Source: CAD feature listing. Evaluate the final solid. Frame: model axes, mm. A direction names the side the tool comes from. Coordinates: 2 decimals unless noted, no trailing zeros. Write each loop counter-clockwise with the first axis right and the second up, starting at its lowest first coordinate (ties: lowest second). Pieces come first, ordered by that corner, then holes. Notation, with made-up numbers: (83, -8.75) - (139, -8.75) arc R31 ccw to (139, 21.25) - close; hole circle Ø7 at (28, -32.5). An arc over 180 degrees is marked (long way). One line per question, with ' | ' between items.
Autodesk Inventor part; units mm, degrees
ref_plane "YZ Plane" through (0, 0, 0) normal (1, 0, 0) x (0, 1, 0)
ref_plane "XZ Plane" through (0, 0, 0) normal (0, 1, 0) x (-1, 0, 0)
ref_plane "XY Plane" through (0, 0, 0) normal (0, 0, 1) x (1, 0, 0)
ref_plane "Plano de trabalho1" through (0, -45, 0) normal (0, 0, 1) x (1, 0, 0)
sketch "Esboço1" plane through (0, -45, 0) normal (0, 0, 1) x (1, 0, 0)
  arc A0 (5.5, 37.5) -> (7.5, 39.5) centre (5.5, 39.5) ccw
  line L0 (7.5, 39.5) -> (7.5, 50.5)
  arc A1 (7.5, 50.5) -> (5.5, 52.5) centre (5.5, 50.5) ccw
  line L1 (5.5, 52.5) -> (-5.5, 52.5)
  arc A2 (-5.5, 52.5) -> (-7.5, 50.5) centre (-5.5, 50.5) ccw
  line L2 (-7.5, 50.5) -> (-7.5, 39.5)
  arc A3 (-7.5, 39.5) -> (-5.5, 37.5) centre (-5.5, 39.5) ccw
  line L3 (-5.5, 37.5) -> (5.5, 37.5)
  circle A4 centre (0, 45) radius 2.1
  arc A5 (-7.5, -5.5) -> (-5.5, -7.5) centre (-5.5, -5.5) ccw
  line L4 (-5.5, -7.5) -> (5.5, -7.5)
  arc A6 (5.5, -7.5) -> (7.5, -5.5) centre (5.5, -5.5) ccw
  line L5 (7.5, -5.5) -> (7.5, 5.5)
  arc A7 (7.5, 5.5) -> (5.5, 7.5) centre (5.5, 5.5) ccw
  line L6 (5.5, 7.5) -> (-5.5, 7.5)
  arc A8 (-5.5, 7.5) -> (-7.5, 5.5) centre (-5.5, 5.5) ccw
  line L7 (-7.5, 5.5) -> (-7.5, -5.5)
  circle A9 centre (0, 0) radius 2.1
  line L8 (7.5, 39.5) -> (7.5, 5.5)
  line L9 (-7.5, 39.5) -> (-7.5, 5.5)
extrude "Extrusão1" add sketch "Esboço1" along normal blind 4
sketch "Esboço2" plane through (0, -45, 4) normal (0, 0, 1) x (1, 0, 0)
  line L0 (7.5, -5.5) -> (7.5, 50.5)
  line L1 (-7.5, 50.5) -> (-7.5, -5.5)
  line L2 (7.5, 24) -> (-7.5, 24)
  line L3 (-7.5, 24) -> (-7.5, 21)
  line L4 (-7.5, 21) -> (7.5, 21)
  line L5 (7.5, 21) -> (7.5, 24)
  line L6 (5.5, 52.5) -> (-5.5, 52.5)
  line L7 (-5.5, -7.5) -> (5.5, -7.5)
  circle A0 centre (0, 32) radius 2.1
  circle A1 centre (0, 13) radius 2.1
  point P0 (0, 45)
  point P1 (7.5, 21)
  dimension "d4" = 28.5
  dimension "d5" = 28.5
  dimension "d6" = 3
  dimension "d7" = 4.2
  dimension "d8" = 4.2
  dimension "d9" = 8
  dimension "d10" = 8
extrude "Extrusão2" cut sketch "Esboço2" against normal blind 1.5
sketch "Esboço3" plane through (0, -13, 2.5) normal (0, 0, 1) x (1, 0, 0)
  circle A0 centre (0, 0) radius 2.1
  circle A1 centre (0, -19) radius 2.1
  point P0 (0, 13)
extrude "Extrusão3" cut sketch "Esboço3" against normal blind 10
fillet "Arredondamento1" radius 1.5 2 edges at (0, -21, 2.5) (0, -24, 2.5)
equation "\"d5\" = d4"
equation "\"d10\" = d9"
properties part number "suporte_termopar_al"
Item 1: Access query for faces 5 (the face through (0, -7, 4)), 6 (the face through (0.11, -23.57, 2.95)). Directions: +Z, -Z, +X, -X, +Y, -Y. A direction counts if a zero-diameter tool reaches every point of the face in a straight line with its end or side. Return the directions, or none.
Check sheet entries:
face 5: +Z, +X, -X, +Y, -Y | face 6: +Z, +X, -X
Item 2: Pin query (flat end, axial travel): pin 1 Ø5 at (x, y) = (0, -45) entering from -Z; pin 2 Ø2.5 at (x, y) = (0, -32) entering from -Z. Return the tip coordinate at first contact, or that it passes through.
Check sheet entries:
pin 1: z = 0 | pin 2: through
Item 3: Cut plane A-A on x = 0. State how many separate pieces and enclosed holes the cut face has, and give its area (3 significant figures).
Check sheet entries:
separate pieces: 5 | enclosed holes: 0 | area: 169 mm²
Item 4: Cut plane B-B on y = -45. Return loops of the section in (x, z).
Check sheet entries:
outline: (-7.5, 0) - (-2.1, 0) - (-2.1, 4) - (-7.5, 4) - close; (2.1, 0) - (7.5, 0) - (7.5, 4) - (2.1, 4) - close
Item 5: Ray query, line 1 along Y through (x, z) = (0, 2.3); line 2 along Y through (x, z) = (-6.25, 3.2); line 3 along Y through (x, z) = (-0.5, 3.85). Return the intervals inside material, ascending. Write a range as [from, to].
Check sheet entries:
line 1: [-52.5, -47.1], [-42.9, -34.1], [-29.9, -15.1], [-10.9, -2.1], [2.1, 7.5] | line 2: [-52.35, -23.77], [-21.23, 7.35] | line 3: [-52.5, -47.04], [-42.96, -34.04], [-29.96, -23.99], [-21.01, -15.04], [-10.96, -2.04], [2.04, 7.5]
Item 6: Cut plane C-C on z = 1.7. Return loops of the section in (x, y), and give its area (3 significant figures).
Check sheet entries:
outline: (-7.5, -50.5) arc R2 ccw to (-5.5, -52.5) - (5.5, -52.5) arc R2 ccw to (7.5, -50.5) - (7.5, 5.5) arc R2 ccw to (5.5, 7.5) - (-5.5, 7.5) arc R2 ccw to (-7.5, 5.5) - close; hole circle Ø4.2 at (0, -45); hole circle Ø4.2 at (0, -32); hole circle Ø4.2 at (0, -13); hole circle Ø4.2 at (0, 0) | area: 841 mm²
Item 7: Cut plane D-D on y = -14. Return loops of the section in (x, z).
Check sheet entries:
outline: (-7.5, 0) - (-1.85, 0) - (-1.85, 4) - (-7.5, 4) - close; (1.85, 0) - (7.5, 0) - (7.5, 4) - (1.85, 4) - close
Item 8: Mould query, pull axis X, two halves, no side actions, for faces 1 (the face through (-0.46, -34.05, 2.03)), 2 (the face through (-0.273, -10.918, 2.028)), 3 (the face through (7.5, -23, 2)), 4 (the face through (-0.11, -21.43, 2.95)). Classes: pulls with the +X half, pulls with the -X half, needs draft (parallel to the pull), parting line crosses it, or undercut.
Check sheet entries:
face 1: undercut | face 2: undercut | face 3: pulls with the +X half | face 4: needs draft
